Drawing for the job (mm, zero at the part's lowest x, y, z). Give positions to 0.01 mm unless a question says otherwise; leave off trailing zeros. Order: outer loops, then holes, each group sorted by start corner. A loop starts at its lowest first (then second) coordinate and runs counter-clockwise, first axis right, second up. Notation, with made-up numbers: (36.25, 24) - (84.25, 24) arc R27 cw to (84.25, 52) - close; hole circle Ø3 at (23, 68). An arc over 180 degrees is marked (long way). One line per item, written item: value.
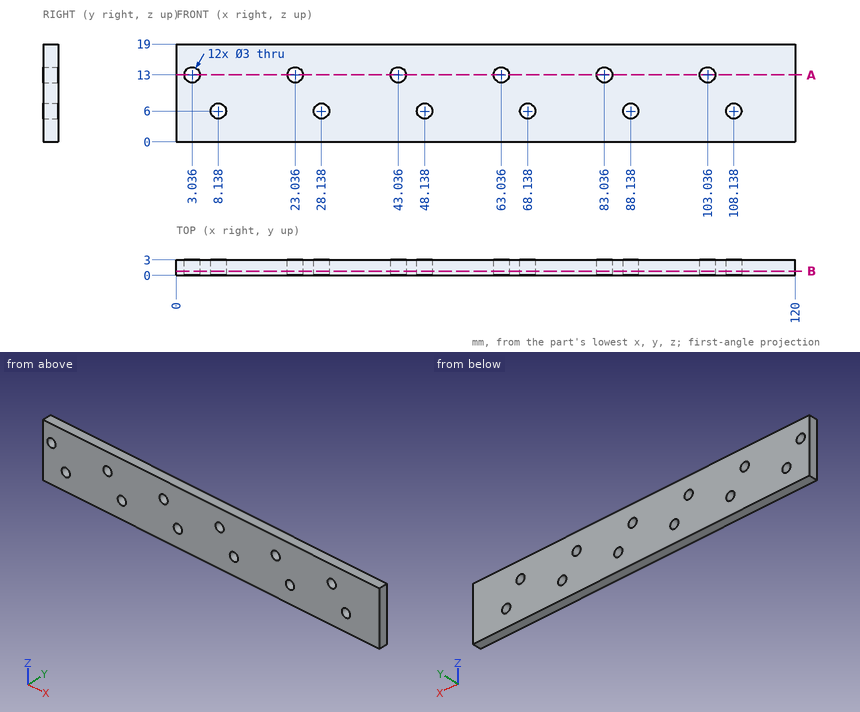
(1) Pin check, flat tip, straight feed: P1, Ø2.5, axis at x = 3.04, z = 13, coming from the +Y side. Stop position of the tip, or through.
Completed:
P1: through
(2) Drill centre lines: line 1 (Z direction, x = 63, y = 0.5); line 2 (Z direction, x = 7, y = 2.65) (1 decimal). Where is each one in solid material? Low to high.
Completed:
line 1: 0 to 11.5, 14.5 to 19
line 2: 0 to 5, 7 to 19
(3) Slice it at B-B, the plane y = 0.85. Count the separate pieces of the cut face and the enclosed holes in it.
Completed:
separate pieces: 1
enclosed holes: 12
(4) Slice it at A-A, the plane z = 13. Give the cut face in (x, y), and give its area (3 significant figures).
Completed:
outline: (0, 0) - (1.54, 0) - (1.54, 3) - (0, 3) - close; (4.54, 0) - (21.54, 0) - (21.54, 3) - (4.54, 3) - close; (24.54, 0) - (41.54, 0) - (41.54, 3) - (24.54, 3) - close; (44.54, 0) - (61.54, 0) - (61.54, 3) - (44.54, 3) - close; (64.54, 0) - (81.54, 0) - (81.54, 3) - (64.54, 3) - close; (84.54, 0) - (101.54, 0) - (101.54, 3) - (84.54, 3) - close; (104.54, 0) - (120, 0) - (120, 3) - (104.54, 3) - close
area: 306 mm²
